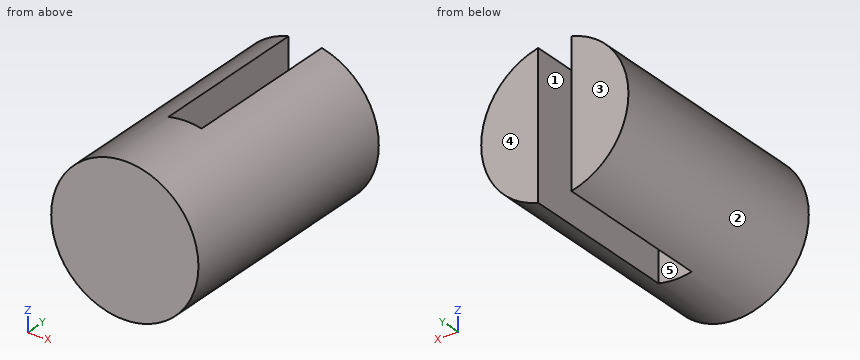
from build123d import *

# Parameters (mm, degrees)
BOSS_EXTRUDE1_DEPTH = 6.35
BOSS_EXTRUDE2_START = 6.35
BOSS_EXTRUDE2_DEPTH = 12.7


with BuildPart() as part:
    # Sketch1 → Boss-Extrude1 (new body)
    with BuildSketch(Plane(origin=(0, 0, 0), x_dir=(1, 0, 0), z_dir=(0, 1, 0))):
        with BuildLine():
            ThreePointArc((-1.27, 5.480885075), (-5.6261, 0), (-1.27, -5.480885075))
            Line((-1.27, -5.480885075), (-1.27, 5.480885075))
        make_face()
        with BuildLine():
            ThreePointArc((-1.27, -5.480885075), (-0.639137568, -5.589678379), (2.1e-08, -5.6261))
            ThreePointArc((2.1e-08, -5.6261), (0.639137588, -5.589678377), (1.27, -5.480885075))
            Line((1.27, -5.480885075), (1.27, 5.480885075))
            ThreePointArc((1.27, 5.480885075), (0.639137578, 5.589678378), (0, 5.6261))
            ThreePointArc((0, 5.6261), (-0.639137578, 5.589678378), (-1.27, 5.480885075))
            Line((-1.27, 5.480885075), (-1.27, -5.480885075))
        make_face()
        with BuildLine():
            Line((1.27, 5.480885075), (1.27, -5.480885075))
            ThreePointArc((1.27, -5.480885075), (4.404438001, -3.50056097), (5.6261, 0))
            ThreePointArc((5.6261, 0), (4.404438001, 3.50056097), (1.27, 5.480885075))
        make_face()
    extrude(amount=BOSS_EXTRUDE1_DEPTH)

    # Sketch1<3> → Boss-Extrude2 (add)
    with BuildSketch(Plane(origin=(0, 0, 0), x_dir=(1, 0, 0), z_dir=(0, 1, 0)).offset(BOSS_EXTRUDE2_START)):
        with BuildLine():
            ThreePointArc((-1.27, 5.480885075), (-5.6261, 0), (-1.27, -5.480885075))
            Line((-1.27, -5.480885075), (-1.27, 5.480885075))
        make_face()
        with BuildLine():
            Line((1.27, 5.480885075), (1.27, -5.480885075))
            ThreePointArc((1.27, -5.480885075), (4.404438001, -3.50056097), (5.6261, 0))
            ThreePointArc((5.6261, 0), (4.404438001, 3.50056097), (1.27, 5.480885075))
        make_face()
    extrude(amount=BOSS_EXTRUDE2_DEPTH)


solid = part.part
Source: CAD feature listing. Evaluate the final solid. Frame: model axes, mm. Face numbers are marked on the shaded views. A direction names the side the tool comes from. Round coordinates to 2 decimals unless told otherwise and drop trailing zeros. Order: outer loops, then holes, each group sorted by start corner. A loop starts at its lowest first (then second) coordinate and runs counter-clockwise, first axis right, second up. Notation, with made-up numbers: (58.5, 45.25) - (110.5, 45.25) arc R20 ccw to (110.5, 70.25) - close; hole circle Ø11 at (18, 65.5). An arc over 180 degrees is marked (long way). Use a Markdown table: item, result. Add a question column.
1. Set-up query: the marked faces 4 and 5. Return all of +Z, -Z, +X, -X, +Y, -Y with unobstructed straight access to the full face (end or side cutting, diameter ignored); none if empty.
2. Section query B-B (y = 14.25). Return the cut outline in (x, z).
3. First-contact query: pin 1 (2 mm diameter, centred on x = -4, y = 6, fed in from -Z); pin 2 (3 mm diameter, centred on x = 3.5, y = 7.5, fed in from +Z); pin 3 (2 mm diameter, centred on y = 15.5, z = -3, fed in from -X). Flat tips, straight axial feed; report the tip coordinate or a pass-through.
4. Line query: probe 1 along X at (y, z) = (6.5, -1.25); probe 2 along X at (y, z) = (13.75, -3.75); probe 3 along Z at (x, y) = (1.25, 4.25). Output: solid intervals per line, ascending.
5. Section query C-C (x = 0). Return the cut outline in (y, z).
6. Mould query, pull axis X, two halves, no side actions, for the marked faces 1, 2 and 3. Classes: +X half, -X half, draft (parallel to the pull), parting line (faces both ways), or undercut.
7. Section query A-A (z = 0). Return the cut outline in (x, y), then the cut area to 3 significant figures.
8. Section query D-D (y = 1.75). Return the cut outline in (x, z), then the cut area to 3 significant figures.
Derived:
| question | item | result |
|---|---|---|
| 1 | face 4 | +Z, -Z, +X, -X, +Y |
| 1 | face 5 | +Z, -Z, +Y |
| 2 | outline | (-1.27, -5.48) - (-1.27, 5.48) arc R5.63 ccw to start; (1.27, -5.48) arc R5.63 ccw to (1.27, 5.48) - close |
| 3 | pin 1 | z = -4.76 |
| 3 | pin 2 | z = 5.26 |
| 3 | pin 3 | x = -5.26 |
| 4 | probe 1 | -5.49 to -1.27, 1.27 to 5.49 |
| 4 | probe 2 | -4.19 to -1.27, 1.27 to 4.19 |
| 4 | probe 3 | -5.49 to 5.49 |
| 5 | outline | (0, -5.63) - (6.35, -5.63) - (6.35, 5.63) - (0, 5.63) - close |
| 6 | face 1 | undercut |
| 6 | face 2 | parting line |
| 6 | face 3 | draft |
| 7 | outline | (-5.63, 0) - (5.63, 0) - (5.63, 19.05) - (1.27, 19.05) - (1.27, 6.35) - (-1.27, 6.35) - (-1.27, 19.05) - (-5.63, 19.05) - close |
| 7 | area | 182 mm2 |
| 8 | outline | circle Ø11.25 at (0, 0) |
| 8 | area | 99.4 mm2 |
